Source: CAD feature listing. Evaluate the final solid. Frame: model axes, mm. A direction names the side the tool comes from. Coordinates: 2 decimals unless noted, no trailing zeros. Write each loop counter-clockwise with the first axis right and the second up, starting at its lowest first coordinate (ties: lowest second). Pieces come first, ordered by that corner, then holes. Notation, with made-up numbers: (47, 65) - (75, 65) arc R14 ccw to (75, 91) - close; hole circle Ø7 at (47.5, 76.5). An arc over 180 degrees is marked (long way). One line per question, with ' | ' between items.
Autodesk Inventor part; units mm, degrees
ref_plane "YZ Plane" through (0, 0, 0) normal (1, 0, 0) x (0, 1, 0)
ref_plane "XZ Plane" through (0, 0, 0) normal (0, 1, 0) x (-1, 0, 0)
ref_plane "XY Plane" through (0, 0, 0) normal (0, 0, 1) x (1, 0, 0)
sketch "Boceto1" plane through (0, 0, 0) normal (0, 0, 1) x (1, 0, 0)
  line L0 (-0.534, 0.5518) -> (14.466, 0.5518)
  line L1 (14.466, 0.5518) -> (14.466, -14.4482)
  line L2 (14.466, -14.4482) -> (-0.534, -14.4482)
  line L3 (-0.534, -14.4482) -> (-0.534, 0.5518)
  line L4 (0.966, -0.9482) -> (12.966, -0.9482)
  line L5 (12.966, -0.9482) -> (12.966, -12.9482)
  line L6 (12.966, -12.9482) -> (0.966, -12.9482)
  line L7 (0.966, -12.9482) -> (0.966, -0.9482)
  point P0 (0, 0)
  point P1 (6.966, -0.9482)
  dimension "d0" = 15
  dimension "d1" = 15
  dimension "d2" = 1.5
  dimension "d3" = 1.5
  dimension "d4" = 1.5
  dimension "d5" = 1.5
extrude "Extrusión1" add sketch "Boceto1" along normal blind 298.4
sketch "Boceto2" plane through (14.466, -14.4482, 0) normal (1, 0, 0) x (0, 0, -1)
  circle A0 centre (-174.2, 7.5) radius 2
  circle A1 centre (-124.2, 7.5) radius 2
  line L0 (0, 0) -> (-298.4, 0)
  line L1 (0, 0) -> (0, 15)
  point P0 (0, 14.4482)
  dimension "d8" = 4
  dimension "d9" = 4
  dimension "d10" = 7.5
  dimension "d11" = 7.5
  dimension "d12" = 50
  dimension "d13" = 124.2
extrude "Extrusión2" cut sketch "Boceto2" against normal blind 10
sketch "Boceto3" plane through (-0.534, -14.4482, 0) normal (-1, 0, 0) x (0, 0, 1)
  circle A0 centre (99.2, 7.5) radius 2
  circle A1 centre (199.2, 7.5) radius 2
  line L0 (0, 15) -> (0, 0)
  point P0 (0, 14.4482)
  dimension "d16" = 4
  dimension "d17" = 4
  dimension "d18" = 100
  dimension "d19" = 99.2
extrude "Extrusión3" cut sketch "Boceto3" against normal blind 10
properties part number "S_horizontal"
Item 1: Access query for faces 4 (the face through (14.466, -7, 147)), 5 (the face through (12.966, -7, 147)). Directions: +Z, -Z, +X, -X, +Y, -Y. A direction counts if a zero-diameter tool reaches every point of the face in a straight line with its end or side. Return the directions, or none.
Check sheet entries:
face 4: +Z, -Z, +X, +Y, -Y | face 5: +Z, -Z
Item 2: Pin query (flat end, axial travel): pin 1 Ø3.5 at (y, z) = (-6.95, 99.2) entering from -X. Return the tip coordinate at first contact, or that it passes through.
Check sheet entries:
pin 1: x = 12.97
Item 3: Cut plane A-A on x = 7.25. Return loops of the section in (y, z).
Check sheet entries:
outline: (-14.45, 0) - (-12.95, 0) - (-12.95, 298.4) - (-14.45, 298.4) - close; (-0.95, 0) - (0.55, 0) - (0.55, 298.4) - (-0.95, 298.4) - close
Item 4: Mould query, pull axis Y, two halves, no side actions, for faces 1 (the face through (7, -14.448, 147)), 2 (the face through (0.966, -7, 147)), 3 (the face through (-0.534, -7, 147)). Classes: pulls with the +Y half, pulls with the -Y half, needs draft (parallel to the pull), parting line crosses it, or undercut.
Check sheet entries:
face 1: pulls with the -Y half | face 2: undercut | face 3: needs draft
Item 5: Cut plane B-B on z = 26. Return loops of the section in (x, y), and give its area (3 significant figures).
Check sheet entries:
outline: (-0.53, -14.45) - (14.47, -14.45) - (14.47, 0.55) - (-0.53, 0.55) - close; hole (0.97, -12.95) - (12.97, -12.95) - (12.97, -0.95) - (0.97, -0.95) - close | area: 81.0 mm²
Item 6: Ray query, line 1 along X through (y, z) = (-7.75, 283.5); line 2 along Y through (x, z) = (0.4, 99.2); line 3 along Y through (x, z) = (5.75, 199.5). Return the intervals inside material, ascending. Write a range as [from, to].
Check sheet entries:
line 1: [-0.53, 0.97], [12.97, 14.47] | line 2: [-14.45, -8.95], [-4.95, 0.55] | line 3: [-14.45, -12.95], [-0.95, 0.55]
